```python
from build123d import *

# Parameters (mm, degrees)
SKETCH1_R           = 11
BOSS_EXTRUDE1_DEPTH = 20
SKETCH2_R           = 3.25
CUT_EXTRUDE1_DEPTH  = 20
SKETCH3_R           = 6.7
CUT_EXTRUDE2_DEPTH  = 19
SKETCH5_R           = 10
CUT_EXTRUDE3_DEPTH  = 7


with BuildPart() as part:
    # Sketch1 → Boss-Extrude1 (new body)
    with BuildSketch(Plane(origin=(0, 0, 0), x_dir=(1, 0, 0), z_dir=(0, 1, 0))):
        with Locations(Location((0, 0, 0), (0, 0, 270))):
            Circle(SKETCH1_R)
    extrude(amount=BOSS_EXTRUDE1_DEPTH)

    # Sketch2 → Cut-Extrude1 (cut)
    with BuildSketch(Plane(origin=(0, 0, 0), x_dir=(1, 0, 0), z_dir=(0, 1, 0))):
        with Locations(Location((0, 0, 0), (0, 0, 270))):
            Circle(SKETCH2_R)
    extrude(amount=CUT_EXTRUDE1_DEPTH, mode=Mode.SUBTRACT)

    # Sketch3 → Cut-Extrude2 (cut)
    with BuildSketch(Plane(origin=(0, 20, 0), x_dir=(1, 0, 0), z_dir=(0, 1, 0))):
        with Locations(Location((0, 0, 0), (0, 0, 270))):
            Circle(SKETCH3_R)
    extrude(amount=-CUT_EXTRUDE2_DEPTH, mode=Mode.SUBTRACT)

    # Sketch5 → Cut-Extrude3 (cut)
    with BuildSketch(Plane(origin=(0, 20, 0), x_dir=(1, 0, 0), z_dir=(0, 1, 0))):
        with Locations(Location((0, 0, 0), (0, 0, 270))):
            Circle(SKETCH5_R)
    extrude(amount=-CUT_EXTRUDE3_DEPTH, mode=Mode.SUBTRACT)


solid = part.part
```
The model under review builds one solid part; all positions refer to its coordinate system, in mm. A direction names the side the tool comes from. Round coordinates to 2 decimals unless told otherwise and drop trailing zeros. Loops run counter-clockwise (first coordinate to the right, second up) from the corner with the lowest first, then second, coordinate; pieces in that order, holes last. Notation, with made-up numbers: (-14, 23.25) - (7, 23.25) arc R20 cw to (7, 52.25) - close; hole circle Ø1 at (63, 73.5). An arc over 180 degrees is marked (long way). Write each question's results on one line, items separated by ' | '. Start each with the question number.
Q1. Take a section at A-A on z = 0. Give the boundary of the cut face in (x, y).
Q2. Take a section at B-B on x = 0. Give the boundary of the cut face in (y, z), plus the area to 3 significant figures.
Q3. Take a section at C-C on y = 14.25. Give the boundary of the cut face in (x, z).
Q4. Tool access review of faces 4 (the cylindrical face through (-9.76, 16.55, -2.17)), 5 (the flat face through (-2, 0, -3)): name each direction out of +Z, -Z, +X, -X, +Y, -Y from which nothing blocks a thin tool from reaching the whole face with its end or side.
Q5. Insertion check: P1, Ø10, axis at x = 1, z = 1.5, coming from the +Y side; P2, Ø6, axis at x = -8.5, y = 4, coming from the -Z side; P3, Ø4, axis at x = -3, z = 2, coming from the +Y side; P4, Ø1, axis at x = 2.5, z = 0.5, coming from the +Y side. Each pin has a flat end and moves straight along its axis. Give the tip position at first contact, or say it passes through.
Q6. Wall thickness on line 1 along X through (y, z) = (0.2, 0); line 2 along X through (y, z) = (7.5, 0); line 3 along Y through (x, z) = (-3.5, -7.75): over which ranges is each line inside the solid? List them lowest first. Write a range as [from, to].
Q7. Take a section at D-D on z = 9.25. Give the boundary of the cut face in (x, y), plus the area to 3 significant figures.
Q8. Draft analysis for pull direction X (two halves, no side actions). For faces 1 (the cylindrical face through (-4.1, 7.1, -5.3)), 2 (the flat face through (-10, 20, 2)), 3 (the cylindrical face through (-10.74, 9.86, -2.38)), state which applies: pulls with the +X half, pulls with the -X half, needs draft (parallel to the pull), parting line crosses it, or undercut.
Data:
1) outline: (-11, 0) - (-3.25, 0) - (-3.25, 1) - (-6.7, 1) - (-6.7, 13) - (-10, 13) - (-10, 20) - (-11, 20) - close; (3.25, 0) - (11, 0) - (11, 20) - (10, 20) - (10, 13) - (6.7, 13) - (6.7, 1) - (3.25, 1) - close
2) outline: (0, -11) - (20, -11) - (20, -10) - (13, -10) - (13, -6.7) - (1, -6.7) - (1, -3.25) - (0, -3.25) - close; (0, 3.25) - (1, 3.25) - (1, 6.7) - (13, 6.7) - (13, 10) - (20, 10) - (20, 11) - (0, 11) - close | area: 133 mm²
3) outline: circle Ø22 at (0, 0); hole circle Ø20 at (0, 0)
4) face 4: +Y | face 5: +Z, -Z, +X, -X, -Y
5) P1: stops at y = 13 | P2: stops at z = -9.53 | P3: stops at y = 1 | P4: passes through
6) line 1: x = [-11, -3.25], [3.25, 11] | line 2: x = [-11, -6.7], [6.7, 11] | line 3: y = [0, 13]
7) outline: (-5.95, 0) - (5.95, 0) - (5.95, 20) - (3.8, 20) - (3.8, 13) - (-3.8, 13) - (-3.8, 20) - (-5.95, 20) - close | area: 185 mm²
8) face 1: undercut | face 2: needs draft | face 3: parting line crosses it
